Build history of the part. All positions in model axes, mm. A direction names the side the tool comes from. Round coordinates to 2 decimals unless told otherwise and drop trailing zeros. Loops run counter-clockwise (first coordinate to the right, second up) from the corner with the lowest first, then second, coordinate; pieces in that order, holes last. Notation, with made-up numbers: (0.25, 54.5) - (59.25, 54.5) arc R15 cw to (59.25, 65.5) - close; hole circle Ø11 at (-10, -8.75). An arc over 180 degrees is marked (long way). Use a Markdown table: item, result.
from build123d import *

# Parameters (mm, degrees)
SKETCH1_W           = 87.5
SKETCH1_H           = 141.3
BOSS_EXTRUDE1_DEPTH = 4
SKETCH1_3_W         = 87.5
SKETCH1_3_H         = 141.3
SKETCH1_3_W_2       = 75.5
SKETCH1_3_H_2       = 129.3
BOSS_EXTRUDE2_DEPTH = 6
BOSS_EXTRUDE3_DEPTH = 10
FILLET2_R           = 2.5


with BuildPart() as part:
    # Sketch1 → Boss-Extrude1 (new body)
    with BuildSketch(Plane(origin=(0, 0, 0), x_dir=(1, 0, 0), z_dir=(0, 1, 0))):
        Rectangle(SKETCH1_W, SKETCH1_H)
    extrude(amount=BOSS_EXTRUDE1_DEPTH)

    # Sketch1<3> → Boss-Extrude2 (add)
    with BuildSketch(Plane(origin=(0, 0, 0), x_dir=(1, 0, 0), z_dir=(0, 1, 0))):
        Rectangle(SKETCH1_3_W, SKETCH1_3_H)
        Rectangle(SKETCH1_3_W_2, SKETCH1_3_H_2, mode=Mode.SUBTRACT)
    extrude(amount=-BOSS_EXTRUDE2_DEPTH)

    # Sketch2 → Boss-Extrude3 (add)
    with BuildSketch(Plane(origin=(0, 4, 0), x_dir=(1, 0, 0), z_dir=(0, 1, 0))):
        Polygon((-43.75, 49.188592066), (-53.75, 22.225), (-53.75, -22.225), (-43.75, -49.188592066), (-43.75, -22.225), (-43.75, -14.605), (-48.75, -14.605), (-48.75, 14.605), (-43.75, 14.605), (-43.75, 22.225), align=None)
        Polygon((53.75, 22.225), (43.75, 22.225), (43.75, 14.605), (48.75, 14.605), (48.75, -14.605), (43.75, -14.605), (43.75, -22.225), (43.75, -49.188592066), (53.75, -22.225), align=None)
        Polygon((43.75, 49.188592066), (43.75, 22.225), (53.75, 22.225), align=None)
    extrude(amount=-BOSS_EXTRUDE3_DEPTH)

    # Fillet2
    fillet2_edges = [part.edges().sort_by_distance(p)[0] for p in [
        (0, 4, 70.65),
        (43.75, 4, -59.919296033),
        (-43.75, 4, 59.919296033),
        (0, 4, -70.65),
        (-48.75, 4, -35.706796033),
        (-53.75, -1, -22.225),
        (-43.75, -1, -49.188592066),
        (-43.75, -1, 49.188592066),
        (-53.75, 4, 0),
        (-48.75, 4, 35.706796033),
        (-48.75, 4, 0),
        (43.75, 4, 59.919296033),
        (43.75, -1, -49.188592066),
        (53.75, 4, 0),
        (53.75, -1, -22.225),
        (48.75, 4, 35.706796033),
        (53.75, -1, 22.225),
        (43.75, -1, 49.188592066),
        (48.75, 4, 0),
        (-43.75, 4, -59.919296033),
        (48.75, 4, -35.706796033),
        (43.75, -1, -70.65),
        (43.75, -1, 70.65),
        (-43.75, -1, 70.65),
        (-43.75, -1, -70.65),
    ]]
    fillet(fillet2_edges, radius=FILLET2_R - 0.0001)  # a hair under: the kernel refuses the full size


solid = part.part
Q1. Cut at B-B, the plane x = 30. List the corners of the cut face in (y, z), plus the area to 3 significant figures.
Results found:
| item | result |
|---|---|
| outline | (-6, -70.65) - (1.5, -70.65) arc R2.5 ccw to (4, -68.15) - (4, 68.15) arc R2.5 ccw to (1.5, 70.65) - (-6, 70.65) - (-6, 64.65) - (0, 64.65) - (0, -64.65) - (-6, -64.65) - close |
| area | 635 mm2 |
Q2. Probe line 1 (X direction, y = -2.25, z = -12); line 2 (X direction, y = -3, z = 15); line 3 (Z direction, x = 31.5, y = -2.25). List the from-to ranges inside material, lowest first.
Results found:
| item | result |
|---|---|
| line 1 | x = -53.75 to -48.75, -43.75 to -37.75, 37.75 to 43.75, 48.75 to 53.75 |
| line 2 | x = -53.75 to -37.75, 37.75 to 53.75 |
| line 3 | z = -70.65 to -64.65, 64.65 to 70.65 |
Q3. Pull direction Z, two halves, no side cores. Call faces 5 (the face through (43.75, -2, 59)), 6 (the face through (48.75, -2, 0)), 7 (the face through (47.977, 3.287, -35.628)): pulls with the +Z half, pulls with the -Z half, needs draft (parallel to the pull), parting line crosses it, or undercut.
Results found:
| item | result |
|---|---|
| face 5 | needs draft |
| face 6 | undercut |
| face 7 | pulls with the -Z half |
Q4. Which spindle directions (+Z, -Z, +X, -X, +Y, -Y) get a long thin tool onto all of the face, cutting with end or side? Do faces 1 (the face through (-1, -3, -64.65)), 2 (the face through (43.75, -2, -59)), 3 (the face through (-43.75, -1, 0)), 4 (the face through (-43.75, -2, 59)). Say none if no direction does.
Results found:
| item | result |
|---|---|
| face 1 | -Y |
| face 2 | -Z, +X, +Y, -Y |
| face 3 | +Y, -Y |
| face 4 | +Z, -X, +Y, -Y |
Q5. Drop flat-ended pins along their axis: pin 1 (4 mm diameter, centred on y = -1.5, z = -62, fed in from -X); pin 2 (22.5 mm diameter, centred on x = 5.5, z = -21, fed in from -Y); pin 3 (6 mm diameter, centred on y = 2, z = -25.5, fed in from -X). Give the stop position or say it passes through.
Results found:
| item | result |
|---|---|
| pin 1 | stops at x = -43.75 |
| pin 2 | stops at y = 0 |
| pin 3 | stops at x = -53.63 |
Q6. Cut at C-C, the plane z = -61.5. List the corners of the cut face in (x, y), plus the area to 3 significant figures.
Results found:
| item | result |
|---|---|
| outline | (-43.75, -6) - (-37.75, -6) - (-37.75, 0) - (37.75, 0) - (37.75, -6) - (43.75, -6) - (43.75, 1.5) arc R2.5 ccw to (41.25, 4) - (-41.25, 4) arc R2.5 ccw to (-43.75, 1.5) - close |
| area | 419 mm2 |
Q7. Cut at A-A, the plane z = -11.5. Count the separate pieces of the cut face and the enclosed holes in it, plus the area to 3 significant figures.
Results found:
| item | result |
|---|---|
| separate pieces | 3 |
| enclosed holes | 0 |
| area | 517 mm2 |
